Autodesk Inventor part; units mm, degrees
ref_plane "YZ Plane" through (0, 0, 0) normal (1, 0, 0) x (0, 1, 0)
ref_plane "XZ Plane" through (0, 0, 0) normal (0, 1, 0) x (-1, 0, 0)
ref_plane "XY Plane" through (0, 0, 0) normal (0, 0, 1) x (1, 0, 0)
sketch "Sketch1" plane through (0, 0, 0) normal (0, 0, 1) x (1, 0, 0)
  line L0 (0, 0) -> (30, 0)
  line L1 (30, 0) -> (30, 4)
  line L2 (30, 4) -> (0, 4)
  line L3 (0, 4) -> (0, 0)
  line L4 (15, 4) -> (11, 4)
  line L5 (15, 4) -> (19, 4)
  line L6 (11, 4) -> (11, 60)
  line L7 (19, 4) -> (19, 60)
  line L8 (11, 60) -> (19, 60)
  circle A0 centre (15, 60) radius 7.5
  circle A1 centre (15, 60) radius 12.5
  arc A2 (11, 48.1573) -> (19, 48.1573) centre (15, 60) ccw
  arc A3 (11, 53.6557) -> (19, 53.6557) centre (15, 60) ccw
  dimension "d0" = 30
  dimension "d1" = 4
  dimension "d2" = 4
  dimension "d3" = 4
  dimension "d5" = 60
  dimension "d6" = 15
  dimension "d7" = 25
extrude "Extrusion1" add sketch "Sketch1" along normal mid plane 12 contours L3 L2 L1 L0 | L6 A1 L7 L2
extrude "Extrusion2" add sketch "Sketch1" along normal mid plane 20 contours A1 L7 A0 L6 | L6 A0 L7 A1
sketch "Sketch2" plane through (19, 4, 6) normal (0, 1, 0) x (1, 0, 0)
  line L0 (0, 12) -> (0, 0)
  line L1 (11, 0) -> (0, 0)
  line L2 (11, 12) -> (11, 0)
  line L3 (0, 12) -> (11, 12)
  line L4 (0, 6) -> (11, 6)
  point P0 (-19, 6)
  point P1 (5.5, 6)
hole "Hole1" at (24.5, 4, 0) direction (0, -1, 0) diameter 3.5 end up to surface
ref_plane "Work Plane1" through (15, 4, -6) normal (-1, 0, 0) x (0, 0, 1)
mirror "Mirror1" about plane through (15, 4, -6) normal (-1, 0, 0) of "Hole1"
equation "\"d2\" = d3"
properties part number "rearSight"
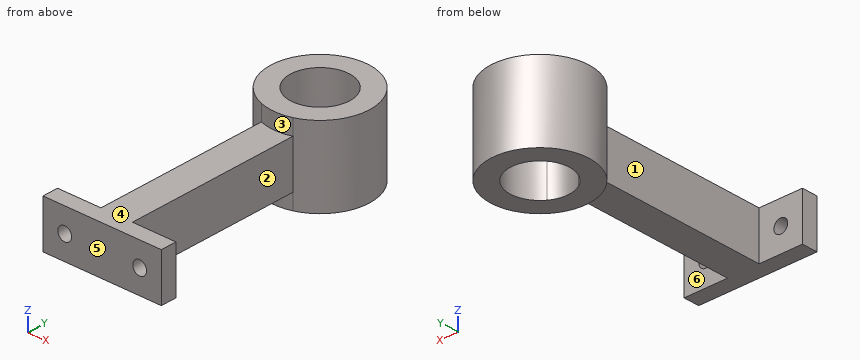
For this review, take the finished solid that the model builds, in its own axes (mm). Face numbers are marked on the shaded views. A direction names the side the tool comes from. Round coordinates to 2 decimals unless told otherwise and drop trailing zeros. Write each loop counter-clockwise with the first axis right and the second up, starting at its lowest first coordinate (ties: lowest second). Pieces come first, ordered by that corner, then holes.
1) Insertion check: pin 1 Ø5.5 at (x, z) = (24.5, 0) entering from +Y; pin 2 Ø3.5 at (x, z) = (3, 2) entering from +Y; pin 3 Ø6 at (x, z) = (4, -7.5) entering from +Y. Each pin has a flat end and moves straight along its axis. Give the tip position at first contact, or say it passes through.
Answer below:
pin 1: stops at y = 70.52
pin 2: stops at y = 67.15
pin 3: stops at y = 69.6
2) Take a section at B-B on x = 15. Give the boundary of the cut face in (y, z).
Answer below:
outline: (0, -6) - (47.5, -6) - (47.5, -10) - (52.5, -10) - (52.5, 10) - (47.5, 10) - (47.5, 6) - (0, 6) - close; (67.5, -10) - (72.5, -10) - (72.5, 10) - (67.5, 10) - close
3) Take a section at C-C on y = 60. Give the boundary of the cut face in (x, z), then the cut area to 3 significant figures.
Answer below:
outline: (2.5, -10) - (7.5, -10) - (7.5, 10) - (2.5, 10) - close; (22.5, -10) - (27.5, -10) - (27.5, 10) - (22.5, 10) - close
area: 200 mm2
4) For line 1 along X through (y, z) = (2.8, 0); line 2 along Z through (x, y) = (24.5, 1.65); line 3 along X through (y, z) = (60, 3.5), list the stretches that pass through material, from the lowest coordinate up.
Answer below:
line 1: x = 0 to 3.75, 7.25 to 22.75, 26.25 to 30
line 2: z = -6 to -1.75, 1.75 to 6
line 3: x = 2.5 to 7.5, 22.5 to 27.5
5) Take a section at A-A on z = 0. Give the boundary of the cut face in (x, y), then the cut area to 3 significant figures.
Answer below:
outline: (0, 0) - (3.75, 0) - (3.75, 4) - (0, 4) - close; (7.25, 0) - (22.75, 0) - (22.75, 4) - (19, 4) - (19, 48.16) arc R12.5 ccw (long way) to (11, 48.16) - (11, 4) - (7.25, 4) - close; (26.25, 0) - (30, 0) - (30, 4) - (26.25, 4) - close; hole circle Ø15 at (15, 60)
area: 756 mm2
6) Machinability: for the marked faces 1, 2 and 3, which of the approach directions +Z, -Z, +X, -X, +Y, -Y give a long, thin tool a straight path to every point of the face, cutting with its end or side? Answer none if there is none.
Answer below:
face 1: +Z, -Z, -X
face 2: +Z, -Z, +X
face 3: +Z, -Y
7) Take a section at D-D on z = -5.25. Give the boundary of the cut face in (x, y), then the cut area to 3 significant figures.
Answer below:
outline: (0, 0) - (30, 0) - (30, 4) - (19, 4) - (19, 48.16) arc R12.5 ccw (long way) to (11, 48.16) - (11, 4) - (0, 4) - close; hole circle Ø15 at (15, 60)
area: 784 mm2
8) Mouldability with a two-part tool opening along Y and no side actions: class the marked faces 4, 5 and 6 as +Y half, -Y half, draft (parallel to the pull), parting line (faces both ways), or undercut.
Answer below:
face 4: draft
face 5: -Y half
face 6: undercut
